from build123d import *

# Parameters (mm, degrees)
F0_R          = 24.432621
F1_DEPTH      = 25.4
F2_R          = 3.310973
F3_DEPTH      = 5.842
F3_DEPTH_BACK = 30.988
F4_COUNT      = 7


with BuildPart() as f1:
    # F0 (on Top) → F1 (new body)
    with BuildSketch(Plane.XY):
        Circle(F0_R)
    extrude(amount=F1_DEPTH)


with BuildPart() as f3:
    # F2 (on face) → F3 (new body, two sides)
    with BuildSketch(Plane.XY.offset(25.4)) as f3_sk:
        with Locations((-9.425403, -22.541401)):
            Circle(F2_R)
    extrude(amount=F3_DEPTH)
    extrude(f3_sk.sketch, amount=-F3_DEPTH_BACK)


with BuildPart() as f4_1:
    # F4: instance of F3
    add(f3.part.rotate(Axis((0, 0, 25.4), (0, 0, 1)), 1 * 360 / F4_COUNT))


with BuildPart() as f4_2:
    # F4: instance of F3
    add(f3.part.rotate(Axis((0, 0, 25.4), (0, 0, 1)), 2 * 360 / F4_COUNT))


with BuildPart() as f4_3:
    # F4: instance of F3
    add(f3.part.rotate(Axis((0, 0, 25.4), (0, 0, 1)), 3 * 360 / F4_COUNT))


with BuildPart() as f4_4:
    # F4: instance of F3
    add(f3.part.rotate(Axis((0, 0, 25.4), (0, 0, 1)), 4 * 360 / F4_COUNT))


with BuildPart() as f4_5:
    # F4: instance of F3
    add(f3.part.rotate(Axis((0, 0, 25.4), (0, 0, 1)), 5 * 360 / F4_COUNT))


with BuildPart() as f4_6:
    # F4: instance of F3
    add(f3.part.rotate(Axis((0, 0, 25.4), (0, 0, 1)), 6 * 360 / F4_COUNT))


with BuildPart() as f1_1:
    add(f1.part)

    # F5: cut F3, F4_1, F4_2, F4_3, F4_4, F4_5, F4_6
    add(f3.part, mode=Mode.SUBTRACT)
    add(f4_1.part, mode=Mode.SUBTRACT)
    add(f4_2.part, mode=Mode.SUBTRACT)
    add(f4_3.part, mode=Mode.SUBTRACT)
    add(f4_4.part, mode=Mode.SUBTRACT)
    add(f4_5.part, mode=Mode.SUBTRACT)
    add(f4_6.part, mode=Mode.SUBTRACT)


solid = f1_1.part
Can you work these out from the model? Positions are in its coordinate system, mm. Coordinates: 2 decimals unless noted, no trailing zeros. Write each loop counter-clockwise with the first axis right and the second up, starting at its lowest first coordinate (ties: lowest second). Pieces come first, ordered by that corner, then holes.
Q1. Imagine slicing it at C-C, the plane y = 15. List the corners of the cut face in (x, z) for me, plus the area to 3 significant figures.
Results found:
outline: (-16.66, 0) - (15.19, 0) - (15.19, 25.4) - (-16.66, 25.4) - close
area: 809 mm2
Q2. Imagine slicing it at B-B, the plane x = 10. List the corners of the cut face in (y, z) for me.
Results found:
outline: (-18.61, 0) - (22.29, 0) - (22.29, 25.4) - (-18.61, 25.4) - close
Q3. For P1, Ø3, axis at x = -2, z = 16, coming from the -Y side; P2, Ø6, axis at y = 19, z = 5, coming from the +X side; P3, Ø3, axis at x = -18.5, z = 12, coming from the -Y side; P4, Ø6, axis at x = 6, y = 8, coming from the -Z side, each with a flat end and sliding along its axis, tell me the tip position at first contact or that it passes through.
Results found:
P1: stops at y = -24.43
P2: stops at x = 15.91
P3: stops at y = -17.55
P4: stops at z = 0
Q4. Please list where these lines run through material, in increasing order: L1, parallel to X at y = 0, z = 5.75; L2, parallel to X at y = 22.5, z = 19.5; L3, parallel to Y at x = 17, z = 7.75.
Results found:
L1: x = -24.43 to 24.43
L2: x = -9.52 to -4, 1.42 to 9.52
L3: y = -17.55 to 13.16
Q5. Imagine slicing it at A-A, the plane z = 9.75. List the corners of the cut face in (x, y) for me.
Results found:
outline: (-24.19, -3.45) arc R3.31 cw to (-22.38, -9.8) arc R24.43 ccw to (-12.39, -21.06) arc R3.31 cw to (-6.29, -23.61) arc R24.43 ccw to (8.74, -22.81) arc R3.31 cw to (14.54, -19.64) arc R24.43 ccw to (23.29, -7.39) arc R3.31 cw to (24.42, -0.88) arc R24.43 ccw to (20.3, 13.6) arc R3.31 cw to (15.91, 18.54) arc R24.43 ccw to (2.02, 24.35) arc R3.31 cw to (-4.58, 24) arc R24.43 ccw to (-17.78, 16.76) arc R3.31 cw to (-21.62, 11.39) arc R24.43 ccw to start
Q6. If we mould it in two halves opening along Y, with no side actions, what happens to faces 1 (the face through (15.75, 14.074, 12.878)), 2 (the face through (-20.297, -5.847, 12.878)), 3 (the face through (-24.055, 4.279, 12.522)), 4 (the face through (0, 0, 25.4))? For each: +Y half, -Y half, draft (parallel to the pull), parting line (faces both ways), or undercut.
Results found:
face 1: undercut
face 2: undercut
face 3: parting line
face 4: draft
